from build123d import *

# Parameters (mm, degrees)
F0_R     = 15.9004
F1_DEPTH = 7.239
F2_R     = 1.89865
F3_DEPTH = 14.479
F6_W     = 3.175
F6_H     = 7.62
F8_R     = 1.27
F9_SIZE  = 0.762
F10_W    = 3.175
F10_H    = 7.0210194136


with BuildPart() as f1:
    # F0 (on Top) → F1 (new body, symmetric)
    with BuildSketch(Plane.XY):
        Circle(F0_R)
    extrude(amount=F1_DEPTH, both=True)

    # F2 (on face) → F3 (cut, through all)
    with BuildSketch(Plane.XY.offset(7.239)):
        Circle(F2_R)
    extrude(amount=-F3_DEPTH, mode=Mode.SUBTRACT)

    # F4 (on Right) → F5 (revolve, cut)
    with BuildSketch(Plane.YZ):
        Polygon((17.7447939179, -4.7117), (17.7447939179, 4.7117), (12.3317, 4.7117), (7.62, 0), (12.3317, -4.7117), align=None)
        Polygon((11.9630908832, 8.8332189437), (5.715, 8.8332189437), (5.715, 2.5851280605), align=None)
        Polygon((5.715, -2.5851280605), (5.715, -8.8332189437), (11.9630908832, -8.8332189437), align=None)
    revolve(axis=Axis((0, 0, 6.9109424949), (0, 0, 1)), mode=Mode.SUBTRACT)

    # F6 (on face) → F7 (join, up to the next surface of F1)
    with BuildSketch(Plane.XY.offset(7.239)):
        with Locations((0, 8.6958226153)):
            Rectangle(F6_W, F6_H)
        Polygon((-11.4031796113, 5.3743139364), (-12.3843085684, 2.3547094971), (-5.1372579143, 0), (-4.1561289571, 3.0196044392), align=None)
        Polygon((-8.6350525796, -9.1843139364), (-6.0664236225, -11.0505321124), (-1.5875, -4.8858226153), (-4.1561289571, -3.0196044392), align=None)
        Polygon((6.0664236225, -11.0505321124), (8.6350525796, -9.1843139364), (4.1561289571, -3.0196044392), (1.5875, -4.8858226153), align=None)
        Polygon((12.3843085684, 2.3547094971), (11.4031796113, 5.3743139364), (4.1561289571, 3.0196044392), (5.1372579143, 0), align=None)
    extrude(until=Until.NEXT, dir=(0, 0, -1))

    # F8
    f8_edges = [f1.edges().sort_by_distance(p)[0] for p in [
        (0, -7.62, 0),
    ]]
    fillet(f8_edges, radius=F8_R)

    # F9
    f9_edges = [f1.edges().sort_by_distance(p)[0] for p in [
        (-15.9004, 0, 7.239),
        (-15.9004, 0, 4.7117),
        (-15.9004, 0, -4.7117),
        (-15.9004, 0, -7.239),
    ]]
    chamfer(f9_edges, length=F9_SIZE)

    # F10 (on face) → F11 (join, up to the next surface of F1)
    with BuildSketch(Plane(origin=(0, 0, -7.239), x_dir=(1, 0, 0), z_dir=(0, 0, -1))):
        with Locations((0, 8.1105777954)):
            Rectangle(F10_W, F10_H)
        Polygon((-3.8843602525, 2.9313014343), (-10.5617465169, 5.1009157509), (-11.542875474, 2.0813113117), (-4.8654892097, -0.088303005), align=None)
        Polygon((-3.9881666606, -2.788424171), (-8.115018328, -8.4685481944), (-5.5463893709, -10.3347663705), (-1.4195377035, -4.654642347), align=None)
        Polygon((1.4195377035, -4.654642347), (5.5463893709, -10.3347663705), (8.115018328, -8.4685481944), (3.9881666606, -2.788424171), align=None)
        Polygon((4.8654892097, -0.088303005), (11.542875474, 2.0813113117), (10.5617465169, 5.1009157509), (3.8843602525, 2.9313014343), align=None)
    extrude(until=Until.NEXT, dir=(0, 0, 1))


solid = f1.part
Input: part model. Units: mm. Frame: model coordinates. A direction names the side the tool comes from. Give positions to 0.01 mm unless a question says otherwise; leave off trailing zeros. Write each loop counter-clockwise with the first axis right and the second up, starting at its lowest first coordinate (ties: lowest second). Pieces come first, ordered by that corner, then holes.
Q1. Section A-A, the plane z = 3.5. Output: boundary loops of the cut face in (x, y) (1 decimal), plus the area to 3 significant figures.
Q2. First-contact query: P1, Ø3.5, axis at y = 9, z = 5.5, coming from the +X side; P2, Ø1, axis at x = -6, z = 1.5, coming from the -Y side; P3, Ø3, axis at x = -7.5, z = 4.5, coming from the +Y side. Flat tips, straight axial feed; report the tip coordinate or a pass-through.
Q3. Set-up query: faces 3 (the face through (-3.45, -15.52, 5.98)), 4 (the face through (3.337, -4.64, -4.945)), 5 (the face through (-1.588, 7, 5)), 6 (the face through (8.55, -1.9, -1.14)). Return all of +Z, -Z, +X, -X, +Y, -Y with unobstructed straight access to the full face (end or side cutting, diameter ignored); none if empty.
Q4. Section C-C, the plane z = 6. Output: boundary loops of the cut face in (x, y) (1 decimal).
Q5. Section B-B, the plane z = -1.5. Output: boundary loops of the cut face in (x, y).
Q6. Pull-direction query (Z, two-part tool) for faces 1 (the face through (11, 6, -4.712)), 2 (the face through (-6.46, -3.77, -5.46)); classes: pulls with the +Z half, pulls with the -Z half, needs draft (parallel to the pull), parting line crosses it, or undercut.
Q7. Material intervals for probe 1 along Z at (x, y) = (7, -11); probe 2 along Y at (x, z) = (2, -4.5); probe 3 along X at (y, z) = (-7, -5.75), sorted ascending.
Filled in:
1. outline: circle Ø22.2 at (0, 0); hole (-6.6, 0.5) arc R6.6 ccw to (-5.1, -4.3) - (-4.5, -3.5) arc R5.7 cw to (-5.7, 0.2) - close; hole (-5.6, 3.5) - (-4.7, 3.2) arc R5.7 cw to (-1.6, 5.5) - (-1.6, 6.4) arc R6.6 ccw to start; hole (-2.5, -6.1) arc R6.6 ccw to (2.5, -6.1) - (1.9, -5.4) arc R5.7 cw to (-1.9, -5.4) - close; hole circle Ø3.8 at (0, 0); hole (1.6, 5.5) arc R5.7 cw to (4.7, 3.2) - (5.6, 3.5) arc R6.6 ccw to (1.6, 6.4) - close; hole (4.5, -3.5) - (5.1, -4.3) arc R6.6 ccw to (6.6, 0.5) - (5.7, 0.2) arc R5.7 cw to start
1. area: 356 mm2
2. P1: stops at x = 14.15
2. P2: stops at y = -7.63
2. P3: stops at y = 14.57
3. face 3: +Z, -Z
3. face 4: -Z
3. face 5: +Z
3. face 6: none
4. outline: circle Ø31.8 at (0, 0); hole (-9, 1.3) arc R9.1 ccw to (-6.6, -6.3) - (-4.5, -3.5) arc R5.7 cw to (-5.7, 0.2) - close; hole (-8.1, 4.3) - (-4.7, 3.2) arc R5.7 cw to (-1.6, 5.5) - (-1.6, 9) arc R9.1 ccw to start; hole (-4, -8.2) arc R9.1 ccw to (4, -8.2) - (1.9, -5.4) arc R5.7 cw to (-1.9, -5.4) - close; hole circle Ø3.8 at (0, 0); hole (1.6, 5.5) arc R5.7 cw to (4.7, 3.2) - (8.1, 4.3) arc R9.1 ccw to (1.6, 9) - close; hole (4.5, -3.5) - (6.6, -6.3) arc R9.1 ccw to (9, 1.3) - (5.7, 0.2) arc R5.7 cw to start
5. outline: circle Ø18.24 at (0, 0); hole circle Ø3.8 at (0, 0)
6. face 1: undercut
6. face 2: needs draft
7. probe 1: z = -7.24 to -4.71, 4.71 to 7.24
7. probe 2: y = -11.95 to -7.36, -5.35 to 5.45, 7.36 to 11.95
7. probe 3: x = -14.28 to -5.46, -1.59 to 1.59, 5.46 to 14.28
